Verification items for this drawing (mm, ordinates from the low corner). Give positions to 0.01 mm unless a question says otherwise; leave off trailing zeros. Order: outer loops, then holes, each group sorted by start corner. A loop starts at its lowest first (then second) coordinate and runs counter-clockwise, first axis right, second up. Notation, with made-up numbers: M -30,67.25 L -23,67.25 A32 cw -23,97.25 Z; hole C 34.25,-11.5 d4. An arc over 180 degrees is marked long. Answer as a JSON object with one key per item and string values.
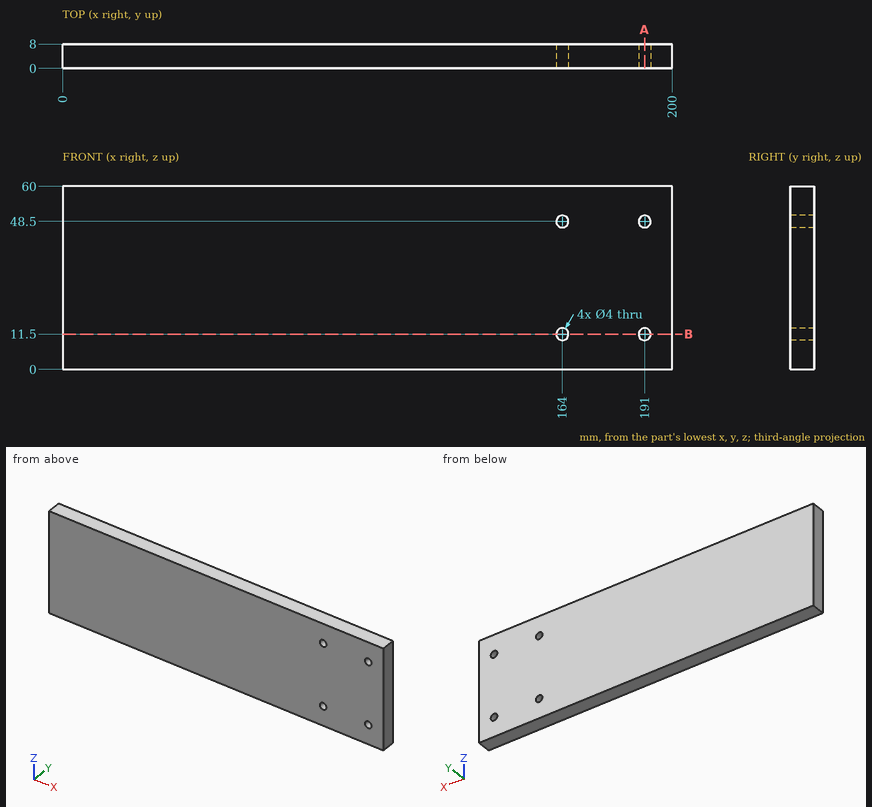
Q1. Section check B-B on z = 11.5. Record the cut outline in (x, y).
Resolved:
{"outline": "M 0,0 L 162,0 L 162,8 L 0,8 Z; M 166,0 L 189,0 L 189,8 L 166,8 Z; M 193,0 L 200,0 L 200,8 L 193,8 Z"}
Q2. Material ranges on L1, parallel to Z at x = 191, y = 6.75; L2, parallel to X at y = 3.5, z = 11.5; L3, parallel to Z at x = 190, y = 5, recorded low to high.
Resolved:
{"L1": "z = 0 to 9.5, 13.5 to 46.5, 50.5 to 60", "L2": "x = 0 to 162, 166 to 189, 193 to 200", "L3": "z = 0 to 9.77, 13.23 to 46.77, 50.23 to 60"}
Q3. Section check A-A on x = 191. Record the cut outline in (y, z).
Resolved:
{"outline": "M 0,0 L 8,0 L 8,9.5 L 0,9.5 Z; M 0,13.5 L 8,13.5 L 8,46.5 L 0,46.5 Z; M 0,50.5 L 8,50.5 L 8,60 L 0,60 Z"}
Q4. Gauge pin test, flat end, axial feed: pin 1 Ø5 at (x, z) = (191, 48.5) entering from +Y. Record the tip position at first contact, or that the pin passes through.
Resolved:
{"pin 1": "stops at y = 8"}
